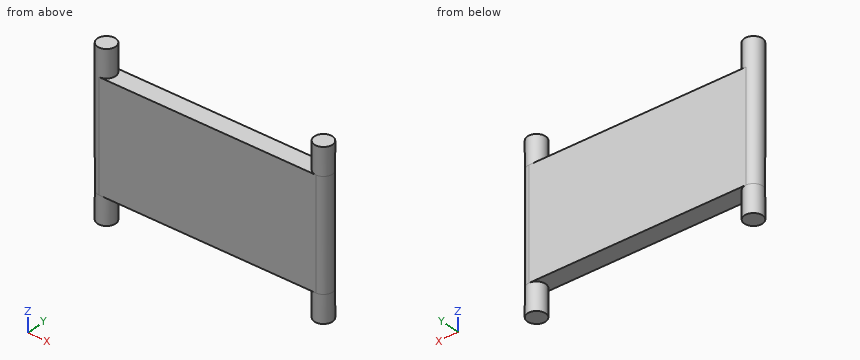
```python
from build123d import *
from build123d.topology import SkipClean

# Parameters (mm, degrees)
BOSS_EXTRUDE1_DEPTH     = 9.525
SKETCH3_R               = 1.5875
BOSS_EXTRUDE3_DEPTH     = 4.7625
MIRROR2_COPY_1_SKETCH_R = 1.5875
MIRROR2_COPY_1_DEPTH    = 4.7625


with BuildPart() as part:
    # Sketch1 → Boss-Extrude1 (new body, symmetric)
    with BuildSketch(Plane.XY):
        with BuildLine():
            Line((-18.82775, 1.5875), (18.82775, 1.5875))
            ThreePointArc((18.82775, 1.5875), (20.41525, 0), (18.82775, -1.5875))
            Line((18.82775, -1.5875), (-18.82775, -1.5875))
            ThreePointArc((-18.82775, -1.5875), (-20.41525, 0), (-18.82775, 1.5875))
        make_face()
    extrude(amount=BOSS_EXTRUDE1_DEPTH, both=True)

    # Sketch3 → Boss-Extrude3 (add)
    with BuildSketch(Plane.XY.offset(9.525)):
        with Locations(Location((-18.82775, 0, 0), (0, 0, 270))):  # turned: the seam where the file's is
            Circle(SKETCH3_R)
    boss_extrude3 = extrude(amount=BOSS_EXTRUDE3_DEPTH)

    # Mirror1: Boss-Extrude3 across plane
    with SkipClean():  # keep this step's faces unmerged: merging them makes the solid invalid here
        add(boss_extrude3.mirror(Plane(origin=(0, 0, 0), x_dir=(0, 0, 1), z_dir=(1, 0, 0))))

    # Mirror2: Boss-Extrude3 across plane
    with SkipClean():  # keep this step's faces unmerged: merging them makes the solid invalid here
        add(boss_extrude3.mirror(Plane.XY))

    # Mirror2 copy 1 sketch → Mirror2 copy 1 (add)
    with BuildSketch(Plane(origin=(0, 0, -9.525), x_dir=(-1, 0, 0), z_dir=(0, 0, -1))):
        with Locations(Location((-18.82775, 0, 0), (0, 0, 270))):  # turned: the seam where the file's is
            Circle(MIRROR2_COPY_1_SKETCH_R)
    extrude(amount=MIRROR2_COPY_1_DEPTH)


solid = part.part
```
Could you check a few things on this model? Use its own coordinates, in mm. Coordinates: 2 decimals unless noted, no trailing zeros. Order: outer loops, then holes, each group sorted by start corner. A loop starts at its lowest first (then second) coordinate and runs counter-clockwise, first axis right, second up. Notation, with made-up numbers: M 23,36.5 L 59,36.5 A23 cw 59,62.5 Z; hole C -34,55.5 d9. An arc over 180 degrees is marked long. Use a Markdown table: item, result. Add a question column.
Q1. I want a section at A-A on z = 10.5. List the corners of the cut face in (x, y) for me (1 decimal).
Q2. I want a section at C-C on x = -10.5. List the corners of the cut face in (y, z) for me (1 decimal).
Q3. I want a section at B-B on y = 0. List the corners of the cut face in (x, z) for me (1 decimal), then the cut area to 3 significant figures.
Q4. I'm going to push flat-ended pins straight in: pin 1 (1.6 mm diameter, centred on x = -2, y = 0, fed in from +Z) (3 decimals); pin 2 (1.5 mm diameter, centred on x = 2, y = -1, fed in from -Z) (3 decimals). Where does each tip first touch, or does it pass through?
Q5. If I drill on L1, parallel to X at y = -0.1, z = 11.75; L2, parallel to Z at x = 9, y = -0.2 (3 decimals); L3, parallel to X at y = 0.8, z = 10.25, over which ranges is the centre line in solid material (lowest first)?
Q6. I want a section at D-D on z = -8. List the corners of the cut face in (x, y) for me (1 decimal), then the cut area to 3 significant figures.
Checked values:
| question | item | result |
|---|---|---|
| 1 | outline | C -18.8,0 d3.2; C 18.8,0 d3.2 |
| 2 | outline | M -1.6,-9.5 L 1.6,-9.5 L 1.6,9.5 L -1.6,9.5 Z |
| 3 | outline | M -20.4,-14.3 L -17.2,-14.3 L -17.2,-9.5 L 17.2,-9.5 L 17.2,-14.3 L 20.4,-14.3 L 20.4,14.3 L 17.2,14.3 L 17.2,9.5 L -17.2,9.5 L -17.2,14.3 L -20.4,14.3 Z |
| 3 | area | 838 mm² |
| 4 | pin 1 | z = 9.525 |
| 4 | pin 2 | z = -9.525 |
| 5 | L1 | -20.41 to -17.24, 17.24 to 20.41 |
| 5 | L2 | -9.525 to 9.525 |
| 5 | L3 | -20.2 to -17.46, 17.46 to 20.2 |
| 6 | outline | M -18.8,-1.6 L 18.8,-1.6 A1.6 ccw 18.8,1.6 L -18.8,1.6 A1.6 ccw Z |
| 6 | area | 127 mm² |
